CAD build for the part. Positions are in the model's coordinates, mm. A direction names the side the tool comes from. Give positions to 0.01 mm unless a question says otherwise; leave off trailing zeros. Loops run counter-clockwise (first coordinate to the right, second up) from the corner with the lowest first, then second, coordinate; pieces in that order, holes last. Notation, with made-up numbers: (-5, 48.25) - (33, 48.25) arc R14 ccw to (33, 56.25) - close; hole circle Ø1 at (61.25, 1.5). An arc over 180 degrees is marked (long way). Return JSON: item names as keys, results as strings.
from build123d import *

# Parameters (mm, degrees)
SKETCH2_W           = 6.21325809
SKETCH2_H           = 30
SKETCH2_R           = 0.7
SKETCH2_R_2         = 2
BOSS_EXTRUDE1_DEPTH = 5
SKETCH3_R           = 3.75
BOSS_EXTRUDE2_DEPTH = 20
SKETCH4_R           = 3
SKETCH4_R_2         = 1.75
BOSS_EXTRUDE3_DEPTH = 6


with BuildPart() as part:
    # Sketch2 → Boss-Extrude1 (new body)
    with BuildSketch(Plane(origin=(0, 0, 0), x_dir=(1, 0, 0), z_dir=(0, 1, 0))):
        with BuildLine():
            Line((16.21325809, 7.5), (16.21325809, 21.207579156))
            Line((16.21325809, 21.207579156), (36.445096698, 32.888436623))
            ThreePointArc((36.445096698, 32.888436623), (36.445096698, 57.535631272), (15.1, 45.212033947))
            Line((15.1, 45.212033947), (15.1, 40))
            Line((15.1, 40), (10, 40))
            Line((10, 40), (10, 45))
            Line((10, 45), (5, 45))
            Line((5, 45), (5, 40))
            Line((5, 40), (0, 40))
            Line((0, 40), (0, -5))
            Line((0, -5), (10, -5))
            Line((10, -5), (10, 0))
            Line((10, 0), (15.1, 0))
            Line((15.1, 0), (15.1, -2.5))
            Line((15.1, -2.5), (40, -2.5))
            ThreePointArc((40, -2.5), (45, 2.5), (40, 7.5))
            Line((40, 7.5), (16.21325809, 7.5))
        make_face()
        with Locations((8.106629045, 20)):
            Rectangle(SKETCH2_W, SKETCH2_H, mode=Mode.SUBTRACT)
        with Locations(Location((19.167389608, 49.421551703, 0), (0, 0, 270))):
            Circle(SKETCH2_R, mode=Mode.SUBTRACT)
        with Locations(Location((30.76585258, 34.306140472, 0), (0, 0, 270))):
            Circle(SKETCH2_R, mode=Mode.SUBTRACT)
        with Locations(Location((29.330064466, 45.212033947, 0), (0, 0, 270))):
            Circle(SKETCH2_R_2, mode=Mode.SUBTRACT)
        with Locations(Location((38.056951209, 51.908409667, 0), (0, 0, 270))):
            Circle(SKETCH2_R, mode=Mode.SUBTRACT)
    extrude(amount=BOSS_EXTRUDE1_DEPTH)

    # Sketch3 → Boss-Extrude2 (add)
    with BuildSketch(Plane(origin=(0, 5, 0), x_dir=(1, 0, 0), z_dir=(0, 1, 0))):
        with Locations(Location((40, 2.5, 0), (0, 0, 270))):
            Circle(SKETCH3_R)
    extrude(amount=-BOSS_EXTRUDE2_DEPTH)

    # Sketch4 → Boss-Extrude3 (add)
    with BuildSketch(Plane(origin=(0, -15, 0), x_dir=(-1, 0, 0), z_dir=(0, -1, 0))):
        with Locations(Location((-40, 2.5, 0), (0, 0, 270))):
            Circle(SKETCH4_R)
        with Locations(Location((-40, 2.5, 0), (0, 0, 90))):
            Circle(SKETCH4_R_2, mode=Mode.SUBTRACT)
    extrude(amount=BOSS_EXTRUDE3_DEPTH)


solid = part.part
1. Cut at C-C, the plane z = -44. Write the cut outline in (x, y), plus the area to 3 significant figures.
Values follow:
{"outline": "(5, 0) - (10, 0) - (10, 5) - (5, 5) - close; (15.1, 0) - (27.74, 0) - (27.74, 5) - (15.1, 5) - close; (30.92, 0) - (43.51, 0) - (43.51, 5) - (30.92, 5) - close", "area": "151 mm²"}
2. Drill centre lines: probe 1 along X at (y, z) = (-19.4, -2.5); probe 2 along X at (y, z) = (0.25, -9.5); probe 3 along Y at (x, z) = (28.5, -50). Where is each one in solid material? Low to high.
Values follow:
{"probe 1": "x = 37 to 38.25, 41.75 to 43", "probe 2": "x = 0 to 5, 11.21 to 16.21", "probe 3": "y = 0 to 5"}
3. Which spindle directions (+Z, -Z, +X, -X, +Y, -Y) get a long thin tool onto all of the face, cutting with end or side? Do faces 4 (the face through (16.213, 2, -14)), 5 (the face through (8, 2, -5)), 6 (the face through (38.29, -17.96, -2.12)), 7 (the face through (8, 2, -45)), 8 (the face through (13, 2, 0)). Say none if no direction does.
Values follow:
{"face 4": "+X, +Y, -Y", "face 5": "+Y, -Y", "face 6": "-Y", "face 7": "-Z, -X, +Y, -Y", "face 8": "+Z, +Y, -Y"}
4. Cut at B-B, the plane x = 9. Write the cut outline in (y, z), plus the area to 3 significant figures.
Values follow:
{"outline": "(0, -45) - (5, -45) - (5, -35) - (0, -35) - close; (0, -5) - (5, -5) - (5, 5) - (0, 5) - close", "area": "100 mm²"}
5. Cut at D-D, the plane z = -2.5. Write the cut outline in (x, y).
Values follow:
{"outline": "(0, 0) - (36.25, 0) - (36.25, -15) - (37, -15) - (37, -21) - (38.25, -21) - (38.25, -15) - (41.75, -15) - (41.75, -21) - (43, -21) - (43, -15) - (43.75, -15) - (43.75, 0) - (45, 0) - (45, 5) - (0, 5) - close"}
6. Pull direction X, two halves, no side cores. Call faces 1 (the face through (5, 2, 5)), 2 (the face through (37.026, -17.958, -2.891)), 3 (the face through (5, 2, -20)): +X half, -X half, draft (parallel to the pull), parting line (faces both ways), or undercut.
Values follow:
{"face 1": "draft", "face 2": "parting line", "face 3": "undercut"}
7. Cut at A-A, the plane z = -20. Write the cut outline in (x, y).
Values follow:
{"outline": "(0, 0) - (5, 0) - (5, 5) - (0, 5) - close; (11.21, 0) - (16.21, 0) - (16.21, 5) - (11.21, 5) - close"}
8. Drop flat-ended pins along their axis: P1, Ø2.5, axis at y = 1.5, z = -16.5, coming from the +X side; P2, Ø2.5, axis at y = 2, z = -43, coming from the -X side; P3, Ø1.5, axis at x = 38.5, y = -11, coming from the +Z side. Give the stop position or say it passes through.
Values follow:
{"P1": "stops at x = 16.21", "P2": "stops at x = 5", "P3": "stops at z = 1.17"}
